Here's how the part is built. I have some questions about the finished solid (model axes, mm). Round coordinates to 2 decimals unless told otherwise and drop trailing zeros. Order: outer loops, then holes, each group sorted by start corner. A loop starts at its lowest first (then second) coordinate and runs counter-clockwise, first axis right, second up. Notation, with made-up numbers: (-10.75, 25.5) - (36.25, 25.5) arc R17 ccw to (36.25, 39.5) - close; hole circle Ø2 at (20, -28.75). An arc over 180 degrees is marked (long way). One line per item, written item: value.
from build123d import *

# Parameters (mm, degrees)
ESQUISSE1_W            = 30
ESQUISSE1_H            = 30
BASE_PLATE_DEPTH       = 2
SKETCH_PERFORATIONS_R  = 0.48
CUT_PERFORATIONS_DEPTH = 10


with BuildPart() as part:
    # Esquisse1 → Base_Plate (new body)
    with BuildSketch(Plane.XY):
        Rectangle(ESQUISSE1_W, ESQUISSE1_H)
    extrude(amount=BASE_PLATE_DEPTH)

    # Sketch_Perforations → Cut_Perforations (cut)
    with BuildSketch(Plane.XY.offset(2)):
        with Locations((-3.41, -10.4)):
            Circle(SKETCH_PERFORATIONS_R)
        with Locations((-3.41, -7.8)):
            Circle(SKETCH_PERFORATIONS_R)
        with Locations((-3.41, -5.2)):
            Circle(SKETCH_PERFORATIONS_R)
        with Locations((-3.41, -2.6)):
            Circle(SKETCH_PERFORATIONS_R)
        with Locations((-3.41, 0)):
            Circle(SKETCH_PERFORATIONS_R)
        with Locations((-3.41, 2.6)):
            Circle(SKETCH_PERFORATIONS_R)
        with Locations((-3.41, 5.2)):
            Circle(SKETCH_PERFORATIONS_R)
        with Locations((-3.41, 7.8)):
            Circle(SKETCH_PERFORATIONS_R)
        with Locations((-3.41, 10.4)):
            Circle(SKETCH_PERFORATIONS_R)
        with Locations((-1.14, -10.4)):
            Circle(SKETCH_PERFORATIONS_R)
        with Locations((-1.14, -7.8)):
            Circle(SKETCH_PERFORATIONS_R)
        with Locations((-1.14, -5.2)):
            Circle(SKETCH_PERFORATIONS_R)
        with Locations((-1.14, -2.6)):
            Circle(SKETCH_PERFORATIONS_R)
        with Locations((-1.14, 0)):
            Circle(SKETCH_PERFORATIONS_R)
        with Locations((-1.14, 2.6)):
            Circle(SKETCH_PERFORATIONS_R)
        with Locations((-1.14, 5.2)):
            Circle(SKETCH_PERFORATIONS_R)
        with Locations((-1.14, 7.8)):
            Circle(SKETCH_PERFORATIONS_R)
        with Locations((-1.14, 10.4)):
            Circle(SKETCH_PERFORATIONS_R)
        with Locations((1.13, -10.4)):
            Circle(SKETCH_PERFORATIONS_R)
        with Locations((1.13, -7.8)):
            Circle(SKETCH_PERFORATIONS_R)
        with Locations((1.13, -5.2)):
            Circle(SKETCH_PERFORATIONS_R)
        with Locations((1.13, -2.6)):
            Circle(SKETCH_PERFORATIONS_R)
        with Locations((1.13, 0)):
            Circle(SKETCH_PERFORATIONS_R)
        with Locations((1.13, 2.6)):
            Circle(SKETCH_PERFORATIONS_R)
        with Locations((1.13, 5.2)):
            Circle(SKETCH_PERFORATIONS_R)
        with Locations((1.13, 7.8)):
            Circle(SKETCH_PERFORATIONS_R)
        with Locations((1.13, 10.4)):
            Circle(SKETCH_PERFORATIONS_R)
        with Locations((3.41, -10.4)):
            Circle(SKETCH_PERFORATIONS_R)
        with Locations((3.41, -7.8)):
            Circle(SKETCH_PERFORATIONS_R)
        with Locations((3.41, -5.2)):
            Circle(SKETCH_PERFORATIONS_R)
        with Locations((3.41, -2.6)):
            Circle(SKETCH_PERFORATIONS_R)
        with Locations((3.41, 0)):
            Circle(SKETCH_PERFORATIONS_R)
        with Locations((3.41, 2.6)):
            Circle(SKETCH_PERFORATIONS_R)
        with Locations((3.41, 5.2)):
            Circle(SKETCH_PERFORATIONS_R)
        with Locations((3.41, 7.8)):
            Circle(SKETCH_PERFORATIONS_R)
        with Locations((3.41, 10.4)):
            Circle(SKETCH_PERFORATIONS_R)
    extrude(amount=-CUT_PERFORATIONS_DEPTH, mode=Mode.SUBTRACT)


solid = part.part
Q1. We'd pull the mould along X, two halves only. Please class faces 1 (the flat face through (0, -15, 1)), 2 (the cylindrical face through (-3.152, 8.205, 1.014)), 3 (the cylindrical face through (1.351, 4.774, 1.014)): released by +X, released by -X, zero draft, split by the parting line, or undercut.
Results list:
face 1: zero draft
face 2: undercut
face 3: undercut
Q2. If we section it at A-A, the plane y = -2.6: Please give me the cut outline in (x, z), then the cut area to 3 significant figures.
Results list:
outline: (-15, 0) - (-3.89, 0) - (-3.89, 2) - (-15, 2) - close; (-2.93, 0) - (-1.62, 0) - (-1.62, 2) - (-2.93, 2) - close; (-0.66, 0) - (0.65, 0) - (0.65, 2) - (-0.66, 2) - close; (1.61, 0) - (2.93, 0) - (2.93, 2) - (1.61, 2) - close; (3.89, 0) - (15, 0) - (15, 2) - (3.89, 2) - close
area: 52.3 mm²
Q3. If I drill on line 1 along X through (y, z) = (10.25, 0.2); line 2 along X through (y, z) = (3, 1.8), over which ranges is the centre line in solid material (lowest first)?
Results list:
line 1: -15 to -3.87, -2.95 to -1.6, -0.68 to 0.67, 1.59 to 2.95, 3.87 to 15
line 2: -15 to -3.68, -3.14 to -1.41, -0.87 to 0.86, 1.4 to 3.14, 3.68 to 15
Q4. If we section it at B-B, the plane x = 1.13: Give the number of separate pieces and of enclosed holes in the cut face, then the cut area to 3 significant figures.
Results list:
separate pieces: 10
enclosed holes: 0
area: 42.7 mm²
